Print and shaded views of the part. All mm, measured from the part's lowest x, y and z. Give positions to 0.01 mm unless a question says otherwise; leave off trailing zeros. Loops run counter-clockwise (first coordinate to the right, second up) from the corner with the lowest first, then second, coordinate; pieces in that order, holes last.
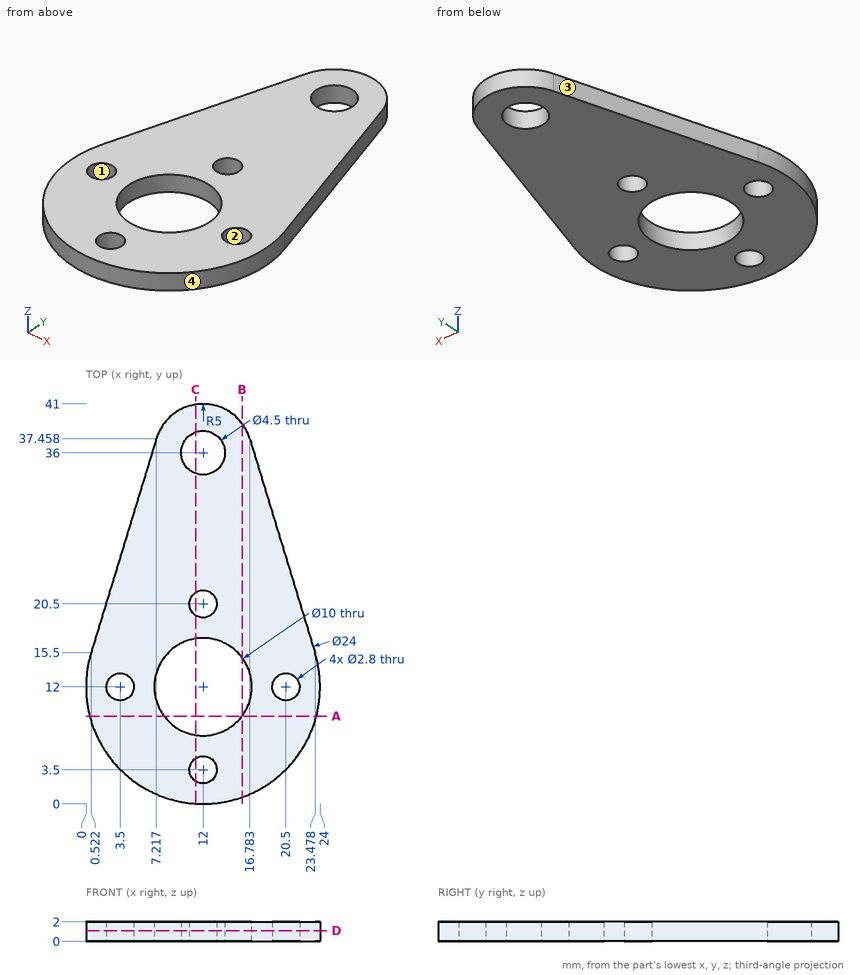
1. Saw through at D-D, the plane z = 1.1. List the corners of the cut face in (x, y).
Responses:
outline: (0.52, 15.5) arc R12 ccw (long way) to (23.48, 15.5) - (16.78, 37.46) arc R5 ccw to (7.22, 37.46) - close; hole circle Ø2.8 at (3.5, 12); hole circle Ø10 at (12, 12); hole circle Ø4.5 at (12, 36); hole circle Ø2.8 at (12, 3.5); hole circle Ø2.8 at (12, 20.5); hole circle Ø2.8 at (20.5, 12)
2. Saw through at C-C, the plane x = 11.25. List the corners of the cut face in (y, z).
Responses:
outline: (0.02, 0) - (2.32, 0) - (2.32, 2) - (0.02, 2) - close; (4.68, 0) - (7.06, 0) - (7.06, 2) - (4.68, 2) - close; (16.94, 0) - (19.32, 0) - (19.32, 2) - (16.94, 2) - close; (21.68, 0) - (33.88, 0) - (33.88, 2) - (21.68, 2) - close; (38.12, 0) - (40.94, 0) - (40.94, 2) - (38.12, 2) - close
3. Pull direction Y, two halves, no side cores. Call the marked faces 1, 2, 3 and 4: released by +Y, released by -Y, zero draft, split by the parting line, or undercut.
Responses:
face 1: undercut
face 2: undercut
face 3: released by +Y
face 4: split by the parting line
4. Drop flat-ended pins along their axis: pin 1 (12 mm diameter, centred on x = 10.5, y = 7, fed in from -Z); pin 2 (1 mm diameter, centred on x = 9, z = 1, fed in from +Y). Give the stop position or say it passes through.
Responses:
pin 1: stops at z = 0
pin 2: stops at y = 40.33
5. Probe line 1 along Y through (x, z) = (13.75, 0.45) (1 decimal); line 2 along Y through (x, z) = (8, 0.25) (1 decimal); line 3 along X through (y, z) = (3, 0.6) (1 decimal). List the from-to ranges inside material, lowest first.
Responses:
line 1: y = 0.1 to 7.3, 16.7 to 34.6, 37.4 to 40.7
line 2: y = 0.7 to 9, 15 to 39
line 3: x = 4.1 to 10.7, 13.3 to 19.9
6. Saw through at B-B, the plane x = 16. List the corners of the cut face in (y, z).
Responses:
outline: (0.69, 0) - (9, 0) - (9, 2) - (0.69, 2) - close; (15, 0) - (39, 0) - (39, 2) - (15, 2) - close
7. Saw through at A-A, the plane y = 9. List the corners of the cut face in (x, z).
Responses:
outline: (0.38, 0) - (8, 0) - (8, 2) - (0.38, 2) - close; (16, 0) - (23.62, 0) - (23.62, 2) - (16, 2) - close
